Design review of the part built by this model. Coordinates are the model's own, in mm. A direction names the side the tool comes from. Give positions to 0.01 mm unless a question says otherwise; leave off trailing zeros. Order: outer loops, then holes, each group sorted by start corner. A loop starts at its lowest first (then second) coordinate and runs counter-clockwise, first axis right, second up. Notation, with made-up numbers: (-36.5, -11.75) -> (2.5, -11.75) arc R22 cw to (2.5, 20.25) -> close; hole circle Ø2 at (26, 89). An arc over 180 degrees is marked (long way). One line per item, written item: value.
from build123d import *

# Parameters (mm, degrees)
F0_R      = 27.5
F1_DEPTH  = 10
F2_R      = 25
F3_DEPTH  = 25
F4_R      = 12
F5_DEPTH  = 15
F6_SIZE   = 1
F9_R      = 12.5
F10_DEPTH = 10
F11_R     = 8.5
F12_DEPTH = 50
F13_R     = 3.175
F14_DEPTH = 20.6


with BuildPart() as f1:
    # F0 (on Front) → F1 (new body)
    with BuildSketch(Plane.XZ):
        Circle(F0_R)
    extrude(amount=F1_DEPTH)

    # F2 (on face) → F3 (join)
    with BuildSketch(Plane.XZ.offset(10)):
        Circle(F2_R)
    extrude(amount=F3_DEPTH)

    # F4 (on face) → F5 (join)
    with BuildSketch(Plane.XZ.offset(35)):
        Circle(F4_R)
    extrude(amount=F5_DEPTH)

    # F6
    f6_edges = [f1.edges().sort_by_distance(p)[0] for p in [
        (-27.5, -10, 0),
        (-27.5, 0, 0),
        (-25, -35, 0),
    ]]
    chamfer(f6_edges, length=F6_SIZE)

    # F7 (on Top) → F8 (revolve, cut)
    with BuildSketch(Plane.XY):
        Polygon((20.75, 0), (0, 0), (0, -20), (15, -20), align=None)
    revolve(axis=Axis((0, -10, 0), (0, -1, 0)), mode=Mode.SUBTRACT)

    # F9 (on face) → F10 (cut)
    with BuildSketch(Plane(origin=(0, -20, 0), x_dir=(-1, 0, 0), z_dir=(0, 1, 0))):
        Circle(F9_R)
    extrude(amount=-F10_DEPTH, mode=Mode.SUBTRACT)

    # F11 (on face) → F12 (join)
    with BuildSketch(Plane.XZ.offset(50)):
        Circle(F11_R)
    extrude(amount=F12_DEPTH)

    # F13 (on face) → F14 (cut)
    with BuildSketch(Plane.XZ.offset(100)):
        Circle(F13_R)
    extrude(amount=-F14_DEPTH, mode=Mode.SUBTRACT)


solid = f1.part
Item 1: Add section B-B on y = -84. Give the boundary of the cut face in (x, z) (3 decimals).
Returned:
outline: circle Ø17 at (0, 0); hole circle Ø6.35 at (0, 0)
Item 2: Draft analysis for pull direction Z (two halves, no side actions). For faces 4 (the flat face through (0, -30, 0)), 5 (the cylindrical face through (-11.99, -42.4, 0.53)), 6 (the conical face through (-3.607, -14.304, -16.242)), 7 (the flat face through (20, -10, 16)), state which applies: pulls with the +Z half, pulls with the -Z half, needs draft (parallel to the pull), parting line crosses it, or undercut.
Returned:
face 4: undercut
face 5: parting line crosses it
face 6: undercut
face 7: needs draft
Item 3: To check wall thickness, follow line 1 along Z through (x, y) = (0, -83.5) (3 decimals); line 2 along Y through (x, z) = (-5.5, 11.5); line 3 along Z through (x, y) = (0, -24.25). State the ranges of each line that lie inside material, in increasing order. Write a range as from..to.
Returned:
line 1: -8.5..-3.175, 3.175..8.5
line 2: -35..-20
line 3: -25..-12.5, 12.5..25
Item 4: Add section D-D on y = -61.5. Give the boundary of the cut face in (x, z).
Returned:
outline: circle Ø17 at (0, 0)
Item 5: Machinability: for faces 1 (the flat face through (3.4, -20, 12.3)), 2 (the flat face through (4, -100, 0)), 3 (the flat face through (-11, -35, 6)), which of the approach directions +Z, -Z, +X, -X, +Y, -Y give a long, thin tool a straight path to every point of the face, cutting with its end or side? Answer none if there is none.
Returned:
face 1: +Y
face 2: +Z, -Z, +X, -X, -Y
face 3: -Y
Item 6: Clearance check with flat-ended pins moving along their axes: P1, Ø9, axis at x = -3, z = -1, coming from the +Y side; P2, Ø3, axis at x = -13, z = -0.5, coming from the +Y side; P3, Ø2, axis at x = -4, z = -11.5, coming from the -Y side. State where each tip first meets the part, or that it passes through.
Returned:
P1: y = -30
P2: y = -20
P3: y = -50
